```python
from build123d import *

# Parameters (mm, degrees)
CROQUIS1_W              = 42
CROQUIS1_H              = 42
SALIENTE_EXTRUIR1_DEPTH = 0.5
CROQUIS2_R              = 1.5
CORTAR_EXTRUIR1_DEPTH   = 0.5
CHAFL_N1_SIZE           = 5


with BuildPart() as part:
    # Croquis1 → Saliente-Extruir1 (new body)
    with BuildSketch(Plane(origin=(0, 0, 0), x_dir=(1, 0, 0), z_dir=(0, 1, 0))):
        with Locations((21, -21)):
            Rectangle(CROQUIS1_W, CROQUIS1_H)
    extrude(amount=SALIENTE_EXTRUIR1_DEPTH)

    # Croquis2 → Cortar-Extruir1 (cut)
    with BuildSketch(Plane(origin=(0, 0.5, 0), x_dir=(1, 0, 0), z_dir=(0, 1, 0))):
        with Locations(Location((5.5, -5.5, 0), (0, 0, 270))):
            Circle(CROQUIS2_R)
        with Locations(Location((36.5, -5.5, 0), (0, 0, 270))):
            Circle(CROQUIS2_R)
        with Locations(Location((36.5, -36.5, 0), (0, 0, 270))):
            Circle(CROQUIS2_R)
        with Locations(Location((5.5, -36.5, 0), (0, 0, 270))):
            Circle(CROQUIS2_R)
    extrude(amount=-CORTAR_EXTRUIR1_DEPTH, mode=Mode.SUBTRACT)

    # Chaflán1
    chafl_n1_edges = [part.edges().sort_by_distance(p)[0] for p in [
        (0, 0.25, 0),
        (42, 0.25, 0),
        (42, 0.25, 42),
        (0, 0.25, 42),
    ]]
    chamfer(chafl_n1_edges, length=CHAFL_N1_SIZE)


solid = part.part
```
For this review, take the finished solid that the model builds, in its own axes (mm). Coordinates: 2 decimals unless noted, no trailing zeros. Loops run counter-clockwise (first coordinate to the right, second up) from the corner with the lowest first, then second, coordinate; pieces in that order, holes last.
1. Add section B-B, the plane z = 36.5. Give the boundary of the cut face in (x, y).
2. Mouldability with a two-part tool opening along Z and no side actions: class faces 1 (the cylindrical face through (5.57, 0.25, 4)), 2 (the flat face through (2.5, 0.2, 2.5)), 3 (the flat face through (21, 0, 21)) as +Z half, -Z half, draft (parallel to the pull), parting line (faces both ways), or undercut.
3. Add section A-A, the plane x = 5.5. Give the boundary of the cut face in (y, z), then the cut area to 3 significant figures.
4. For line 1 (X direction, y = 0.4, z = 36.5); line 2 (X direction, y = 0.25, z = 37), list the stretches that pass through material, from the lowest coordinate up.
5. Insertion check: P1, Ø2.5, axis at x = 36.5, z = 36.5, coming from the -Y side. The pin has a flat end and moves straight along its axis. Give the tip position at first contact, or say it passes through.
Result:
1. outline: (0, 0) - (4, 0) - (4, 0.5) - (0, 0.5) - close; (7, 0) - (35, 0) - (35, 0.5) - (7, 0.5) - close; (38, 0) - (42, 0) - (42, 0.5) - (38, 0.5) - close
2. face 1: undercut
2. face 2: -Z half
2. face 3: draft
3. outline: (0, 0) - (0.5, 0) - (0.5, 4) - (0, 4) - close; (0, 7) - (0.5, 7) - (0.5, 35) - (0, 35) - close; (0, 38) - (0.5, 38) - (0.5, 42) - (0, 42) - close
3. area: 18.0 mm2
4. line 1: x = 0 to 4, 7 to 35, 38 to 42
4. line 2: x = 0 to 4.09, 6.91 to 35.09, 37.91 to 42
5. P1: passes through
